```python
from build123d import *

# Parameters (mm, degrees)
EXTRUDE_START            = 53
SKETCH_3_R               = 8
EXTRUDE_1_DEPTH          = 53
SKETCH_4_W               = 21.869380784
SKETCH_4_H               = 6.809627549
CUT_EXTRUDE_1_DEPTH      = 46
SKETCH_5_R               = 3.5
CUT_EXTRUDE_2_DEPTH      = 70
PATTERN_CIRCULAR_1_COUNT = 6
HOLE_WIZARD_M41_D        = 4.5
HOLE_WIZARD_M41_DEPTH    = 14
HOLE_WIZARD_M41_TIP      = 1.351936393
SKETCH_14_R              = 9.95061624
SKETCH_14_R_2            = 8
CUT_EXTRUDE_5_DEPTH      = 10


with BuildPart() as part:
    # Эскиз2 → Повернуть1 (revolve)
    with BuildSketch(Plane.XY):
        Polygon((-10, 0), (-54, 0), (-62, -18), (-69, -18), (-69, -23), (-63, -23), (-63, -59), (-69, -59), (-69, -64), (-23, -64), (-14, -68), (0, -68), (0, -8), (-8, -8), (-8, -11.730591033), (-10, -11.730591033), align=None)
    revolve(axis=Axis((0, -8, 0), (0, -1, 0)))

    # Эскиз3 → Бобышка-Вытянуть1 (add)
    with BuildSketch(Plane.XZ.offset(68).offset(EXTRUDE_START)):
        with Locations(Location((0, 0, 0), (0, 0, 180))):
            Circle(SKETCH_3_R)
    extrude(amount=-EXTRUDE_1_DEPTH)

    # Эскиз4 → Вырез-Вытянуть1 (cut)
    with BuildSketch(Plane.XZ.offset(121)):
        with Locations((-0.065477188, 8.404813774)):
            Rectangle(SKETCH_4_W, SKETCH_4_H)
    extrude(amount=-CUT_EXTRUDE_1_DEPTH, mode=Mode.SUBTRACT)

    # Эскиз5 → Вырез-Вытянуть2 (cut)
    with BuildSketch(Plane.XZ.offset(121)):
        with Locations(Location((0, 0, 0), (0, 0, 270))):
            Circle(SKETCH_5_R)
    extrude(amount=-CUT_EXTRUDE_2_DEPTH, mode=Mode.SUBTRACT)

    # Эскиз7 → Зенковка для винта с полупотайной головкой M51 (revolve, cut)
    with BuildSketch(Plane(origin=(-1.157683247, -64, -60), x_dir=(0, 0, -1), z_dir=(1, 0, 0))):
        Polygon((0, 0), (0, 15.652366702), (2.75, 14), (2.75, 2.45), (5.2, 0), align=None)
    hole_wizard_m51 = revolve(axis=Axis((-1.157683247, -70.35, -60), (0, 1, 0)), mode=Mode.SUBTRACT)

    # Круговой массив1: Зенковка для винта с полупотайной головкой M51 ×6 about axis
    pattern_circular_1_axis = Axis((0, 0, 0), (0, 1, 0))
    for i in range(1, PATTERN_CIRCULAR_1_COUNT):
        add(hole_wizard_m51.rotate(pattern_circular_1_axis, i * 360 / PATTERN_CIRCULAR_1_COUNT), mode=Mode.SUBTRACT)

    # Отверстие с зазором M41
    with Locations(Plane(origin=(0, -8, 0), x_dir=(1, 0, 0), z_dir=(0, 1, 0))):
        with Locations((0, 0)):
            Hole(HOLE_WIZARD_M41_D / 2, depth=HOLE_WIZARD_M41_DEPTH)
            with Locations((0, 0, -(HOLE_WIZARD_M41_DEPTH + HOLE_WIZARD_M41_TIP / 2))):  # 118° drill point
                Cone(0, HOLE_WIZARD_M41_D / 2, HOLE_WIZARD_M41_TIP, mode=Mode.SUBTRACT)

    # Эскиз14 → Вырез-Вытянуть5 (cut)
    with BuildSketch(Plane.XZ.offset(68)):
        Circle(SKETCH_14_R)
        with Locations(Location((0, 0, 0), (0, 0, 180))):
            Circle(SKETCH_14_R_2, mode=Mode.SUBTRACT)
    extrude(amount=-CUT_EXTRUDE_5_DEPTH, mode=Mode.SUBTRACT)


solid = part.part
```
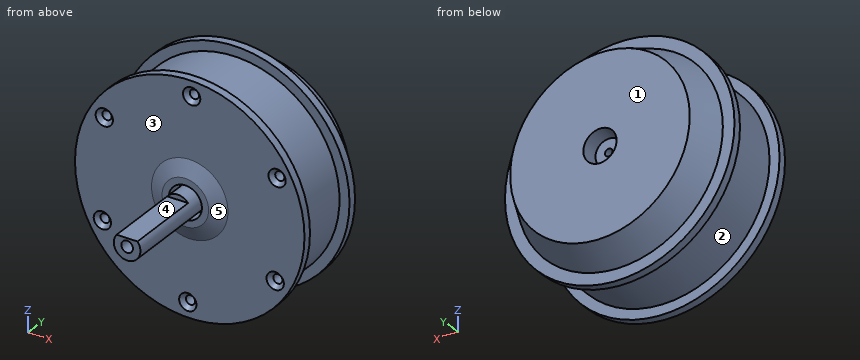
Model file for the job. Use its own axes, mm. Face numbers are marked on the shaded views. A direction names the side the tool comes from. Coordinates: 2 decimals unless noted, no trailing zeros. Loops run counter-clockwise (first coordinate to the right, second up) from the corner with the lowest first, then second, coordinate; pieces in that order, holes last. Notation, with made-up numbers: (22, 31) -> (54, 31) arc R30 cw to (54, 62) -> close; hole circle Ø9 at (-34.5, 52.5). An arc over 180 degrees is marked (long way). Answer as a JSON object with one key per item and string values.
Q1. Pull direction Y, two halves, no side cores. Call the marked faces 1, 2 and 3: released by +Y, released by -Y, zero draft, split by the parting line, or undercut.
Report:
{"face 1": "released by +Y", "face 2": "undercut", "face 3": "released by -Y"}
Q2. Cut at A-A (y = -96). List the corners of the cut face in (x, z) (3 decimals), and give its area (3 significant figures).
Report:
{"outline": "(-6.245, 5) arc R8 ccw (long way) to (6.245, 5) -> close; hole circle Ø7 at (0, 0)", "area": "136 mm2"}
Q3. Flat gauge pins, fed straight in: P1, Ø10, axis at x = -2, z = 35.5, coming from the -Y side; P2, Ø5, axis at x = -1.16, z = -60, coming from the +Y side; P3, Ø6, axis at y = -72.5, z = 4.5, coming from the -X side. Where does each tip first touch, or does it go through?
Report:
{"P1": "stops at y = -64", "P2": "stops at y = -7.9", "P3": "stops at x = -7.86"}
Q4. 3-axis set-ups, long thin cutter, end or side, ignore diameter. For the marked faces 4 and 5: which of +Z, -Z, +X, -X, +Y, -Y reach the whole face in a straight line?
Report:
{"face 4": "+Z, +X, -X, -Y", "face 5": "-Y"}
Q5. Probe probe 1 along Y at (x, z) = (48, 43.5); probe 2 along Y at (x, z) = (6, -4); probe 3 along X at (y, z) = (-52, -29). List the from-to ranges inside material, lowest first.
Report:
{"probe 1": "y = -64 to -59, -23 to -18", "probe 2": "y = -121 to -8", "probe 3": "x = -55.93 to -55.29, -49.79 to 49.5, 53.27 to 55.93"}
